```python
from build123d import *

# Parameters (mm, degrees)
F1_DEPTH = 7.5
F2_R     = 2.974485
F3_DEPTH = 33.760661
F4_R     = 2.974485
F5_DEPTH = 10.938791


with BuildPart() as f1:
    # F0 (on Front) → F1 (new body, symmetric)
    with BuildSketch(Plane.XZ):
        Polygon((5.826252, 12.139047), (6.064818, 26.734496), (3.536387, 26.734496), (1.821829, 26.267877), (0.454524, 25.215268), (-0.413607, 23.500709), (-0.413607, 14.103194), (-0.771711, 12.139047), (-2.855225, 9.263365), (-5.937089, 6.604715), (-8.137005, 3.577773), (-10.042827, 0), (-10.937791, -4.908744), (-10.937791, -8.619478), (-10.042827, -12.583584), (-8.289473, -16.242759), (-5.937089, -20.206865), (-4.16116, -22.265492), (-4.16116, -26.83912), (11.410935, -26.83912), (11.410935, -22.188919), (6.728393, -22.188919), (2.381469, -21.396385), (0.454524, -20.130632), (-3.029408, -17.767416), (-4.477831, -14.718102), (-5.937089, -11.211392), (-7.069747, -7.09482), (-6.673481, -4.921359), (-6.069345, -1.607767), (-4.325366, 1.748186), (-1.733449, 5.10243), (0.454524, 6.989942), (3.297916, 8.304209), (5.279969, 9.14277), align=None)
        Polygon((16.093477, -22.188919), (11.410935, -22.188919), (11.410935, -26.83912), (26.98303, -26.83912), (26.98303, -22.265492), (28.758958, -20.206865), (31.111343, -16.242759), (32.864696, -12.583584), (33.759661, -8.619478), (33.759661, -4.908744), (32.864696, 0), (30.958875, 3.577773), (28.758958, 6.604715), (25.677094, 9.263365), (23.593581, 12.139047), (23.235477, 14.103194), (23.235477, 23.500709), (22.367346, 25.215268), (21.00004, 26.267877), (19.285482, 26.734496), (16.757051, 26.734496), (16.995617, 12.139047), (17.5419, 9.14277), (19.523954, 8.304209), (22.367346, 6.989942), (24.555319, 5.10243), (27.147235, 1.748186), (28.891215, -1.607767), (29.495351, -4.921359), (29.891617, -7.09482), (28.758958, -11.211392), (27.2997, -14.718102), (25.851278, -17.767416), (22.367346, -20.130632), (20.440401, -21.396385), align=None)
    extrude(amount=F1_DEPTH, both=True)

    # F2 (on Right) → F3 (cut, through all)
    with BuildSketch(Plane.YZ):
        with Locations((0.075872, 18.351913)):
            Circle(F2_R)
    extrude(amount=F3_DEPTH, mode=Mode.SUBTRACT)

    # F4 (on face) → F5 (cut, through all)
    with BuildSketch(Plane.YZ):
        with Locations((0.075872, 18.351913)):
            Circle(F4_R)
    extrude(amount=-F5_DEPTH, mode=Mode.SUBTRACT)


solid = f1.part
```
Input: part model. Units: mm. Frame: model coordinates. A direction names the side the tool comes from. Round coordinates to 2 decimals unless told otherwise and drop trailing zeros. Order: outer loops, then holes, each group sorted by start corner. A loop starts at its lowest first (then second) coordinate and runs counter-clockwise, first axis right, second up. Notation, with made-up numbers: (-2.75, 19.25) - (50.25, 19.25) arc R22 ccw to (50.25, 57.25) - close; hole circle Ø2 at (88, 42.5). An arc over 180 degrees is marked (long way). Answer in a Markdown table with one row per item.
Item 1: Mould query, pull axis Z, two halves, no side actions, for faces 4 (the flat face through (20.926, -0.105, 7.656)), 5 (the flat face through (28.04, -0.11, -12.94)), 6 (the flat face through (23.235, -2, 21)), 7 (the flat face through (21.693, -0.105, 25.734)). Classes: released by +Z, released by -Z, zero draft, split by the parting line, or undercut.
Model answer:
| item | result |
|---|---|
| face 4 | undercut |
| face 5 | undercut |
| face 6 | zero draft |
| face 7 | released by +Z |
Item 2: Section query D-D (x = 8). Return the cut outline in (y, z), then the cut area to 3 significant figures.
Model answer:
| item | result |
|---|---|
| outline | (-7.5, -26.84) - (7.5, -26.84) - (7.5, -22.19) - (-7.5, -22.19) - close |
| area | 69.8 mm² |
Item 3: Reachability of faces 1 (the flat face through (-3.743, -0.105, -16.264)), 2 (the flat face through (-0.414, -2, 21)), 3 (the flat face through (33.306, -0.105, -10.629)) from +Z, -Z, +X, -X, +Y, -Y: full face, straight path, thin tool, end or side. Return the list, or none.
Model answer:
| item | result |
|---|---|
| face 1 | +Y, -Y |
| face 2 | +Z, -X, +Y, -Y |
| face 3 | -Z, +X, +Y, -Y |
Item 4: Section query A-A (z = -3). Return the cut outline in (x, y), then the cut area to 3 significant figures.
Model answer:
| item | result |
|---|---|
| outline | (-10.59, -7.5) - (-6.32, -7.5) - (-6.32, 7.5) - (-10.59, 7.5) - close; (29.15, -7.5) - (33.41, -7.5) - (33.41, 7.5) - (29.15, 7.5) - close |
| area | 128 mm² |
Item 5: Section query C-C (y = -1.5). Give the number of separate pieces and of enclosed holes in the cut face, then the cut area to 3 significant figures.
Model answer:
| item | result |
|---|---|
| separate pieces | 3 |
| enclosed holes | 0 |
| area | 619 mm² |
Item 6: Section query B-B (z = -9.5). Return the cut outline in (x, y).
Model answer:
| item | result |
|---|---|
| outline | (-10.74, -7.5) - (-6.41, -7.5) - (-6.41, 7.5) - (-10.74, 7.5) - close; (29.23, -7.5) - (33.56, -7.5) - (33.56, 7.5) - (29.23, 7.5) - close |
Item 7: Line query: line 1 (X direction, y = -0.75, z = -24); line 2 (X direction, y = 6, z = 11); line 3 (Z direction, x = 15, y = -3). Output: solid intervals per line, ascending.
Model answer:
| item | result |
|---|---|
| line 1 | x = -4.16 to 26.98 |
| line 2 | x = -1.6 to 5.62, 17.2 to 24.42 |
| line 3 | z = -26.84 to -22.19 |
Item 8: Pin query (flat end, axial travel): pin 1 (4.5 mm diameter, centred on x = 10.5, y = -2.5, fed in from +Z); pin 2 (2 mm diameter, centred on y = -5, z = -10.5, fed in from -X); pin 3 (4.5 mm diameter, centred on y = 2, z = 19.5, fed in from -X). Return the tip coordinate at first contact, or that it passes through.
Model answer:
| item | result |
|---|---|
| pin 1 | stops at z = -22.19 |
| pin 2 | stops at x = -10.74 |
| pin 3 | stops at x = -0.41 |
